Could you check a few things on this model? Use its own coordinates, in mm. A direction names the side the tool comes from. Round coordinates to 2 decimals unless told otherwise and drop trailing zeros. Loops run counter-clockwise (first coordinate to the right, second up) from the corner with the lowest first, then second, coordinate; pieces in that order, holes last. Notation, with made-up numbers: (37, 18) -> (89, 18) arc R23 cw to (89, 47) -> close; hole circle Ø8 at (13, -12.5). An arc over 180 degrees is marked (long way). Put each result on its own line as item: value. Start each with the question number.
1. If we mould it in two halves opening along Y, with no side actions, what happens to faces 1 (the conical face through (0, 56.1, -3.8)), 2 (the cylindrical face through (2.1, 50.6, -3.8)), 3 (the cylindrical face through (4.5, 52.2, -2.5))? For each: pulls with the +Y half, pulls with the -Y half, needs draft (parallel to the pull), parting line crosses it, or undercut.
2. Imagine slicing it at A-A, the plane y = 24.5. Please give me the cut outline in (x, z).
3. Which directions (+Z, -Z, +X, -X, +Y, -Y) give clear straight access to the entire face, cutting with the end or side of a thin tool? Please do faces 4 (the cylindrical face through (2.1, 53.8, -3.8)), 5 (the cylindrical face through (0.1, 56.9, -1.8)), 6 (the cylindrical face through (0, 2.9, 0.5)), 7 (the flat face through (2, 28.1, -3.5)), 8 (the flat face through (-1.5, 29.7, 0.5)).
4. I'm going to push flat-ended pins straight in: P1, Ø0.5, axis at y = 38, z = 0.5, coming from the +X side; P2, Ø0.6, axis at x = 2, y = 51.5, coming from the +Z side; P3, Ø1.7, axis at y = 28.5, z = -2, coming from the +X side. Where does each tip first touch, or does it pass through?
5. I need wall thicknesses on line 1 (X direction, y = 54.4, z = -0.2); line 2 (Y direction, x = -4.1, z = -0.5); line 3 (X direction, y = 49.5, z = -2.3). Which ranges of each line are inside material? Lowest first, please. Write a range as [from, to].
Autodesk Inventor part; units mm, degrees
ref_plane "YZ Plane" through (0, 0, 0) normal (1, 0, 0) x (0, 1, 0)
ref_plane "XZ Plane" through (0, 0, 0) normal (0, 1, 0) x (-1, 0, 0)
ref_plane "XY Plane" through (0, 0, 0) normal (0, 0, 1) x (1, 0, 0)
sketch "Sketch1" plane through (0, 0, 0) normal (0, 0, 1) x (1, 0, 0)
  line L0 (0, 54.4) -> (0, 4.4) construction
  line L1 (-1.5, 54.4) -> (-1.5, 4.4)
  line L2 (1.5, 4.4) -> (1.5, 54.4)
  arc A0 (1.5, 54.4) -> (-1.5, 54.4) centre (0, 54.4) ccw
  arc A1 (-1.5, 4.4) -> (1.5, 4.4) centre (0, 4.4) ccw
  line L3 (-5.6, 4.4) -> (-5.6, 54.4)
  line L4 (5.6, 54.4) -> (5.6, 4.4)
  line L5 (-4.1, 4.4) -> (-4.1, 54.4)
  arc A2 (4.1, 54.4) -> (-4.1, 54.4) centre (0, 54.4) ccw
  line L6 (4.1, 54.4) -> (4.1, 4.4)
  arc A3 (-4.1, 4.4) -> (4.1, 4.4) centre (0, 4.4) ccw
  line L7 (-2.5, 4.4) -> (-2.5, 54.4)
  arc A4 (2.5, 54.4) -> (-2.5, 54.4) centre (0, 54.4) ccw
  line L8 (2.5, 54.4) -> (2.5, 4.4)
  arc A5 (-2.5, 4.4) -> (2.5, 4.4) centre (0, 4.4) ccw
  arc A6 (5.6, 54.4) -> (3.4641, 58.8) centre (0, 54.4) ccw
  arc A7 (-3.4641, 58.8) -> (-5.6, 54.4) centre (0, 54.4) ccw
  arc A8 (-5.6, 4.4) -> (-3.4641, 0) centre (0, 4.4) ccw
  arc A9 (3.4641, 0) -> (5.6, 4.4) centre (0, 4.4) ccw
  line L9 (-3.4641, 0) -> (3.4641, 0)
  line L10 (-3.4641, 58.8) -> (3.4641, 58.8)
  point P0 (0, 0)
  point P1 (0, 1.5)
  point P2 (0, 29.4)
  point P3 (4.1, 29.4)
  point P4 (-4.1, 29.4)
  dimension "d0" = 3
  dimension "d1" = 50
  dimension "d2" = 4.1
  dimension "d3" = 2.6
  dimension "d4" = 1
extrude "Extrusion1" add sketch "Sketch1" along normal blind 1 contours A0 L2 A1 L1
extrude "Extrusion2" add sketch "Sketch1" against normal blind 4 contours A0 L2 A1 L1 | L7 A4 L8 A5
extrude "Extrusion3" add sketch "Sketch1" against normal blind 0.6 contours L3 A7 L10 A6 L4 A9 L9 A8 | L5 A2 L6 A3
chamfer "Chamfer1" distance 1 angle 45 4 edges at (2.5, 29.4, -4) (0, 1.9, -4) (-2.5, 29.4, -4) (0, 56.9, -4)
hole "Hole1" at (-4.1, 29.4, 0) at (4.1, 29.4, 0) at (-4.1, 54.4, 0) at (4.1, 54.4, 0) at (4.1, 4.4, 0) at (-4.1, 4.4, 0) direction (0, 0, -1) diameter 1.6 depth 8 tip angle 118
sketch "Sketch2" plane through (2.5, 4.4, -0.6) normal (1, 0, 0) x (0, 0, -1)
  line L0 (2.4, 50) -> (2.4, 0)
  line L1 (0, 50) -> (2.4, 50)
  line L2 (0, 50) -> (0, 0)
  line L3 (0, 0) -> (2.4, 0)
  line L4 (2.4, 48.8) -> (2.4, 46.8) construction
  line L5 (1.9, 48.8) -> (1.9, 46.8)
  line L6 (2.9, 46.8) -> (2.9, 48.8)
  arc A0 (2.9, 48.8) -> (1.9, 48.8) centre (2.4, 48.8) ccw
  arc A1 (1.9, 46.8) -> (2.9, 46.8) centre (2.4, 46.8) ccw
  line L7 (1.4, 48.8) -> (1.4, 46.8)
  arc A2 (1.4, 46.8) -> (3.4, 46.8) centre (2.4, 46.8) ccw
  line L8 (3.4, 46.8) -> (3.4, 48.8)
  arc A3 (3.4, 48.8) -> (1.4, 48.8) centre (2.4, 48.8) ccw
  circle A4 centre (2.4, 48.8) radius 0.5
  circle A5 centre (2.4, 46.8) radius 0.5
  circle A6 centre (2.4, 47.8) radius 0.5
  point P0 (-0.6, -4.4)
  dimension "d21" = 2
  dimension "d22" = 1
  dimension "d23" = 2.4
  dimension "d24" = 0
  dimension "d25" = 1.2
  dimension "d26" = 0.5
  dimension "d27" = 1
  dimension "d29" = 1
extrude "Extrusion4" add sketch "Sketch2" against normal blind 1 contours A3 L8 A2 L0 A1 L6 A0 | L0 A0 L5 A1 A2 L7 A3
extrude "Extrusion5" add sketch "Sketch2" along normal mid plane 8 contours A0 A4 L0 | L0 A4 A0 | A6 L0 | L0 A6 | A5 A1 L0 | L0 A1 A5
properties part number "ASSEMBLY_Regolith_container_level_sensor" material "Aluminum 6061"
Entries:
1. face 1: pulls with the +Y half
1. face 2: pulls with the -Y half
1. face 3: undercut
2. outline: (-5.6, -0.6) -> (-2.5, -0.6) -> (-2.5, -3) -> (-1.5, -4) -> (1.5, -4) -> (2.5, -3) -> (2.5, -0.6) -> (5.6, -0.6) -> (5.6, 0) -> (1.5, 0) -> (1.5, 1) -> (-1.5, 1) -> (-1.5, 0) -> (-5.6, 0) -> close
3. face 4: -Z, +X, +Y
3. face 5: -Z, +Y
3. face 6: +Z, -Y
3. face 7: -Z, +X, -Y
3. face 8: +Z, -X, +Y, -Y
4. P1: x = 1.5
4. P2: z = 0
4. P3: x = 2.5
5. line 1: [-5.6, -4.9], [-3.3, 3.3], [4.9, 5.6]
5. line 2: [0.59, 3.6], [5.2, 28.6], [30.2, 53.6], [55.2, 58.21]
5. line 3: [-2.5, 2.5]
